Read the model definition and answer for the solid it produces. Units are mm, in the model's axes. A direction names the side the tool comes from. Give positions to 0.01 mm unless a question says otherwise; leave off trailing zeros. Order: outer loops, then holes, each group sorted by start corner. A loop starts at its lowest first (then second) coordinate and runs counter-clockwise, first axis right, second up. Notation, with made-up numbers: (70, -17) - (105, -17) arc R24 ccw to (105, 9) - close; hole circle Ø9 at (-34.75, 65). An arc over 180 degrees is marked (long way). One line per item, written item: value. Start each with the question number.
```python
from build123d import *

# Parameters (mm, degrees)
SKETCH015_R     = 4.5
SKETCH015_R_2   = 1.5
PAD008_DEPTH    = 8
SKETCH016_R     = 11
SKETCH016_R_2   = 4.5
PAD009_DEPTH    = 2
SKETCH017_R     = 8
POCKET004_DEPTH = 8.4
CHAMFER003_SIZE = 0.2
FILLET002_R     = 0.4


with BuildPart() as part:
    # Sketch015 → Pad008 (new body)
    with BuildSketch(Plane.XY):
        with BuildLine():
            ThreePointArc((-16.650526, 21), (-18.950462, 18.950462), (-21, 16.650526))
            Line((-21, 16.650526), (-21, -16.650526))
            ThreePointArc((-21, -16.650526), (-18.950462, -18.950462), (-16.650526, -21))
            Line((-16.650526, -21), (16.650526, -21))
            ThreePointArc((16.650526, -21), (18.950462, -18.950462), (21, -16.650526))
            Line((21, 16.650526), (21, -16.650526))
            ThreePointArc((21, 16.650526), (18.950462, 18.950462), (16.650526, 21))
            Line((-16.650526, 21), (16.650526, 21))
        make_face()
        Circle(SKETCH015_R, mode=Mode.SUBTRACT)
        with Locations((-15.5, 15.5)):
            Circle(SKETCH015_R_2, mode=Mode.SUBTRACT)
        with Locations((15.5, 15.5)):
            Circle(SKETCH015_R_2, mode=Mode.SUBTRACT)
        with Locations((15.5, -15.5)):
            Circle(SKETCH015_R_2, mode=Mode.SUBTRACT)
        with Locations((-15.5, -15.5)):
            Circle(SKETCH015_R_2, mode=Mode.SUBTRACT)
    extrude(amount=PAD008_DEPTH)

    # Sketch016 (on Face15 of Pad008) → Pad009 (join)
    with BuildSketch(Plane.XY.offset(8)):
        Circle(SKETCH016_R)
        Circle(SKETCH016_R_2, mode=Mode.SUBTRACT)
    extrude(amount=PAD009_DEPTH)

    # Sketch017 → Pocket004 (cut)
    with BuildSketch(Plane.XY):
        Circle(SKETCH017_R)
    extrude(amount=POCKET004_DEPTH, mode=Mode.SUBTRACT)

    # Chamfer003
    chamfer003_edges = [part.edges().sort_by_distance(p)[0] for p in [
        (-11, 0, 10),
        (14, 15.5, 8),
        (-17, 15.5, 8),
        (-17, -15.5, 8),
        (14, -15.5, 8),
        (-4.5, 0, 10),
        (-4.5, 0, 8.4),
    ]]
    chamfer(chamfer003_edges, length=CHAMFER003_SIZE)

    # Fillet002
    fillet002_edges = [part.edges().sort_by_distance(p)[0] for p in [
        (16.650526, 21, 4),
        (21, 16.650526, 4),
        (21, -16.650526, 4),
        (16.650526, -21, 4),
        (-21, -16.650526, 4),
        (-16.650526, -21, 4),
        (-21, 16.650526, 4),
        (-16.650526, 21, 4),
    ]]
    fillet(fillet002_edges, radius=FILLET002_R)


with BuildPart() as part_1:
    # Body005 placement: moved
    add(part.part.moved(Location((0, 0, 30))))


solid = part_1.part
```
1) Section D-D on z = 31.75 is taken. Write down the section's boundary in (x, y), plus the area to 3 significant figures.
2) Find the intervals of material crossed by probe 1 along Y at (x, z) = (-15.5, 36); probe 2 along X at (y, z) = (15, 35.75); probe 3 along Y at (x, z) = (0, 35), in increasing order. Write a range as from..to.
3) Section A-A on y = -15.5 is taken. Write down the section's boundary in (x, z), plus the area to 3 significant figures.
4) The mould has two halves that part along X. Classify faces 1 (the cylindrical face through (-18.9, 19, 33.9)), 2 (the cylindrical face through (18.9, -19, 33.9)), 3 (the flat face through (9, 0, 30)), 4 (the cylindrical face through (-17, 15.57, 33.85)): +X half, -X half, draft (parallel to the pull), parting line (faces both ways), or undercut.
5) Each of these flat-tipped pins is pushed along its axis until it touches: pin 1 (6 mm diameter, centred on x = 14, y = -11.5, fed in from +Z); pin 2 (2.5 mm diameter, centred on x = 15.5, y = 15.5, fed in from +Z); pin 3 (14.5 mm diameter, centred on x = 0, y = 0, fed in from -Z). Where does it stop, or does it pass through?
6) Section B-B on x = 0 is taken. Write down the section's boundary in (y, z), plus the area to 3 significant figures.
7) For faces 5 (the cylindrical face through (-1.73, -7.81, 34.14)), 6 (the flat face through (9, -9, 38)), 7 (the flat face through (0, 21, 34)), determine the directions among +Z, -Z, +X, -X, +Y, -Y from which every point of the face is accessible in a straight line to the end or side of a thin tool.
Solved:
1. outline: (-21, -16.51) arc R0.4 ccw to (-20.91, -16.76) arc R26.8 ccw to (-16.76, -20.91) arc R0.4 ccw to (-16.51, -21) - (16.51, -21) arc R0.4 ccw to (16.76, -20.91) arc R26.8 ccw to (20.91, -16.76) arc R0.4 ccw to (21, -16.51) - (21, 16.51) arc R0.4 ccw to (20.91, 16.76) arc R26.8 ccw to (16.76, 20.91) arc R0.4 ccw to (16.51, 21) - (-16.51, 21) arc R0.4 ccw to (-16.76, 20.91) arc R26.8 ccw to (-20.91, 16.76) arc R0.4 ccw to (-21, 16.51) - close; hole circle Ø3 at (-15.5, -15.5); hole circle Ø3 at (-15.5, 15.5); hole circle Ø16 at (0, 0); hole circle Ø3 at (15.5, -15.5); hole circle Ø3 at (15.5, 15.5)
1. area: 1,500 mm2
2. probe 1: y = -21..-17, -14..14, 17..21
2. probe 2: x = -21..-16.91, -14.09..14.09, 16.91..21
2. probe 3: y = -21..-8, 8..21
3. outline: (-21, 30) - (-17, 30) - (-17, 37.8) - (-17.2, 38) - (-21, 38) - close; (-14, 30) - (14, 30) - (14, 37.8) - (13.8, 38) - (-13.8, 38) - (-14, 37.8) - close; (17, 30) - (21, 30) - (21, 38) - (17.2, 38) - (17, 37.8) - close
3. area: 288 mm2
4. face 1: -X half
4. face 2: +X half
4. face 3: draft
4. face 4: undercut
5. pin 1: stops at z = 38
5. pin 2: passes through
5. pin 3: stops at z = 38.4
6. outline: (-21, 30) - (-8, 30) - (-8, 38.4) - (-4.7, 38.4) - (-4.5, 38.6) - (-4.5, 39.8) - (-4.7, 40) - (-10.8, 40) - (-11, 39.8) - (-11, 38) - (-21, 38) - close; (4.5, 38.6) - (4.7, 38.4) - (8, 38.4) - (8, 30) - (21, 30) - (21, 38) - (11, 38) - (11, 39.8) - (10.8, 40) - (4.7, 40) - (4.5, 39.8) - close
6. area: 231 mm2
7. face 5: -Z
7. face 6: +Z
7. face 7: +Z, -Z, +X, -X, +Y
